Design review of the part shown in the three views and the two pictorial views. Dimensions are in mm from the part's minimum x, y and z. A direction names the side the tool comes from. Give positions to 0.01 mm unless a question says otherwise; leave off trailing zeros. Loops run counter-clockwise (first coordinate to the right, second up) from the corner with the lowest first, then second, coordinate; pieces in that order, holes last. Notation, with made-up numbers: (30.5, 84.25) -> (77.5, 84.25) arc R18 ccw to (77.5, 118.25) -> close; hole circle Ø9 at (2, 13.25). An arc over 180 degrees is marked (long way). Answer as CSV lines item,"result".
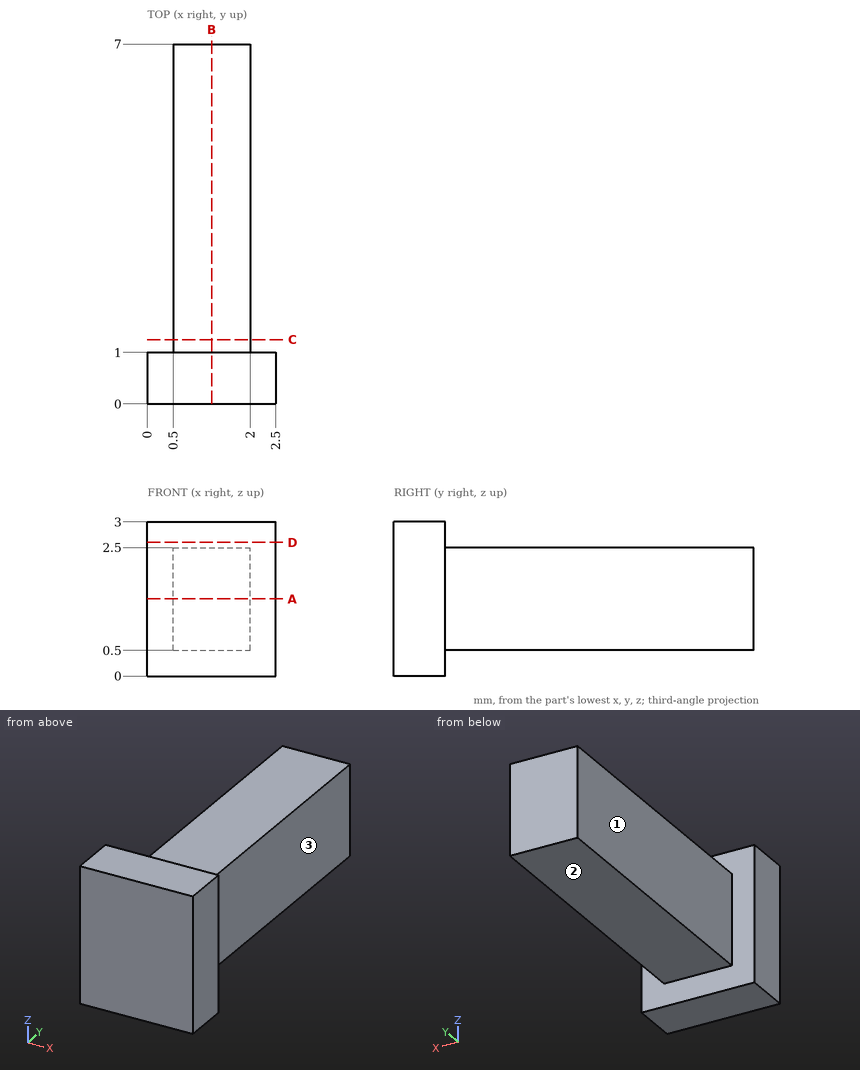
Q1. Clearance check with flat-ended pins moving along their axes: pin 1 Ø1.6 at (y, z) = (5, 1.5) entering from -X; pin 2 Ø0.6 at (y, z) = (5.5, 2) entering from +X. State where each tip first meets the part, or that it passes through.
Filled sheet:
pin 1,"stops at x = 0.5"
pin 2,"stops at x = 2"
Q2. We need section A-A, the plane z = 1.5. State the section outline as (x, y) points.
Filled sheet:
outline,"(0, 0) -> (2.5, 0) -> (2.5, 1) -> (2, 1) -> (2, 7) -> (0.5, 7) -> (0.5, 1) -> (0, 1) -> close"
Q3. For the marked faces 1, 2 and 3, list the 3-axis set-ups (+Z, -Z, +X, -X, +Y, -Y) from which the entire face can be reached by the end or side of a thin tool; tool diameter is ignored.
Filled sheet:
face 1,"+Z, -Z, -X, +Y"
face 2,"-Z, +X, -X, +Y"
face 3,"+Z, -Z, +X, +Y"
Q4. We need section C-C, the plane y = 1.25. State the section outline as (x, z) points.
Filled sheet:
outline,"(0.5, 0.5) -> (2, 0.5) -> (2, 2.5) -> (0.5, 2.5) -> close"
Q5. We need section B-B, the plane x = 1.25. State the section outline as (y, z) points, and give its area (3 significant figures).
Filled sheet:
outline,"(0, 0) -> (1, 0) -> (1, 0.5) -> (7, 0.5) -> (7, 2.5) -> (1, 2.5) -> (1, 3) -> (0, 3) -> close"
area,"15.0 mm^2"
Q6. We need section D-D, the plane z = 2.6. State the section outline as (x, y) points.
Filled sheet:
outline,"(0, 0) -> (2.5, 0) -> (2.5, 1) -> (0, 1) -> close"
Q7. To check wall thickness, follow probe 1 along Z at (x, y) = (1.5, 6.5); probe 2 along Y at (x, z) = (1.45, 0.3); probe 3 along X at (y, z) = (5.25, 0.7). State the ranges of each line that lie inside material, in increasing order. Write a range as from..to.
Filled sheet:
probe 1,"z = 0.5..2.5"
probe 2,"y = 0..1"
probe 3,"x = 0.5..2"
